Source: three-view drawing plus pictorial views. Frame: mm from the lowest corner of the part. Round coordinates to 2 decimals unless told otherwise and drop trailing zeros. Loops run counter-clockwise (first coordinate to the right, second up) from the corner with the lowest first, then second, coordinate; pieces in that order, holes last. Notation, with made-up numbers: M -24.5,83.25 L 9.5,83.25 A9 ccw 9.5,93.25 Z; hole C 80.5,31 d5. An arc over 180 degrees is marked long. Answer as a JSON object with one key per item and string values.
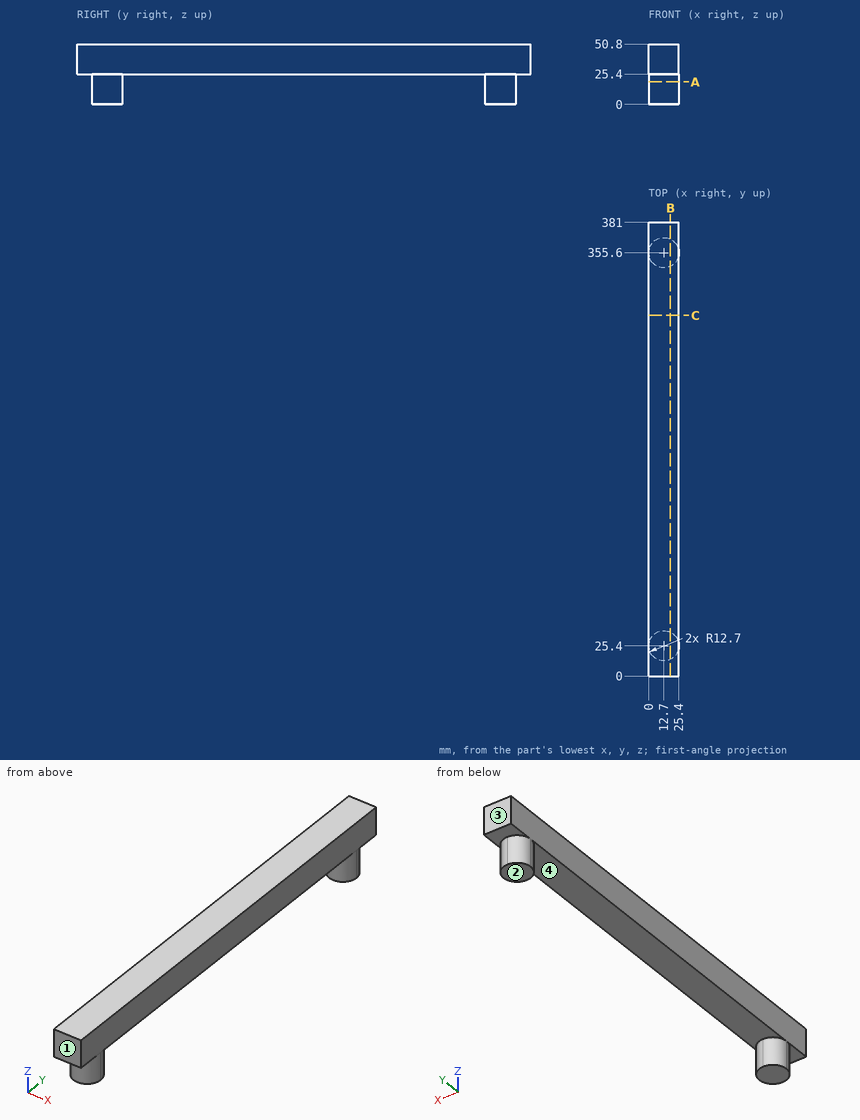
1) Pull-direction query (Y, two-part tool) for the marked faces 1, 2, 3 and 4; classes: +Y half, -Y half, draft (parallel to the pull), parting line (faces both ways), or undercut.
Geometry results:
{"face 1": "-Y half", "face 2": "draft", "face 3": "+Y half", "face 4": "undercut"}
2) Cut plane A-A on z = 19. Return the cut outline in (x, y).
Geometry results:
{"outline": "C 12.7,25.4 d25.4; C 12.7,355.6 d25.4"}
3) Line query: probe 1 along Z at (x, y) = (19.25, 338.5); probe 2 along Y at (x, z) = (2, 6.5); probe 3 along Y at (x, z) = (11.25, 21). Output: solid intervals per line, ascending.
Geometry results:
{"probe 1": "25.4 to 50.8", "probe 2": "18.56 to 32.24, 348.76 to 362.44", "probe 3": "12.78 to 38.02, 342.98 to 368.22"}
4) Cut plane B-B on x = 18.25. Return the cut outline in (y, z), and give its area (3 significant figures).
Geometry results:
{"outline": "M 0,25.4 L 13.98,25.4 L 13.98,0 L 36.82,0 L 36.82,25.4 L 344.18,25.4 L 344.18,0 L 367.02,0 L 367.02,25.4 L 381,25.4 L 381,50.8 L 0,50.8 Z", "area": "10,800 mm2"}
5) Cut plane C-C on y = 303. Return the cut outline in (x, z).
Geometry results:
{"outline": "M 0,25.4 L 25.4,25.4 L 25.4,50.8 L 0,50.8 Z"}
6) First-contact query: pin 1 (4 mm diameter, centred on x = 16.5, y = 60, fed in from -Z); pin 2 (4 mm diameter, centred on x = 13.5, z = 5.5, fed in from -Y). Flat tips, straight axial feed; report the tip coordinate or a pass-through.
Geometry results:
{"pin 1": "z = 25.4", "pin 2": "y = 12.7"}
